The model under review builds one solid part; all positions refer to its coordinate system, in mm. A direction names the side the tool comes from. Round coordinates to 2 decimals unless told otherwise and drop trailing zeros. Order: outer loops, then holes, each group sorted by start corner. A loop starts at its lowest first (then second) coordinate and runs counter-clockwise, first axis right, second up.
```python
from build123d import *

# Parameters (mm, degrees)
SKETCH_1_W                = 42
SKETCH_1_H                = 30
EXTRUDE_1_DEPTH           = 40
CUT_EXTRUDE_1_DEPTH       = 85.059502735
HOLE_WIZARD_1_D           = 5.5
HOLE_WIZARD_1_CBORE_D     = 10
HOLE_WIZARD_1_CBORE_DEPTH = 23
CUT_EXTRUDE_2_DEPTH       = 85.059502735
HOLE_WIZARD_M8_1_D        = 6.8
HOLE_WIZARD_M8_1_DEPTH    = 19.75
HOLE_WIZARD_M8_1_TIP      = 2.042926105


with BuildPart() as part:
    # 草图1 → 凸台-拉伸1 (new, symmetric)
    with BuildSketch(Plane.XY):
        Rectangle(SKETCH_1_W, SKETCH_1_H)
    extrude(amount=EXTRUDE_1_DEPTH, both=True)

    # 草图2 → 切除-拉伸1 (cut, through all)
    with BuildSketch(Plane.XY.offset(40)):
        Polygon((-21, 12), (6, -15), (-21, -15), align=None)
    extrude(amount=-CUT_EXTRUDE_1_DEPTH, mode=Mode.SUBTRACT)

    # 打孔尺寸根据内六角圆柱头螺钉的类型1 (through all)
    with Locations(Plane(origin=(0, -15, 0), x_dir=(-1, 0, 0), z_dir=(0, -1, 0))):
        with Locations((0, -30), (0, 30), (0, 0)):
            CounterBoreHole(HOLE_WIZARD_1_D / 2, HOLE_WIZARD_1_CBORE_D / 2, HOLE_WIZARD_1_CBORE_DEPTH)

    # 草图3 → 切除-拉伸2 (cut, through all)
    with BuildSketch(Plane.XY.offset(40)):
        Polygon((-1.071067812, -7.928932188), (7.414213562, 0.556349186), (22.970562748, -15), (6, -15), align=None)
    extrude(amount=-CUT_EXTRUDE_2_DEPTH, mode=Mode.SUBTRACT)

    # M8 螺纹孔1
    with Locations(Plane(origin=(3.985281374, 3.985281374, 0), x_dir=(-0.7071067811865477, 0.7071067811865474, 0), z_dir=(-0.7071067811865474, -0.7071067811865477, 0))):
        with Locations((-12.849242405, 25), (-12.849242405, -25)):
            Hole(HOLE_WIZARD_M8_1_D / 2, depth=HOLE_WIZARD_M8_1_DEPTH)
            with Locations((0, 0, -(HOLE_WIZARD_M8_1_DEPTH + HOLE_WIZARD_M8_1_TIP / 2))):  # 118° drill point
                Cone(0, HOLE_WIZARD_M8_1_D / 2, HOLE_WIZARD_M8_1_TIP, mode=Mode.SUBTRACT)


solid = part.part
```
(1) Insertion check: pin 1 (8 mm diameter, centred on x = -2, z = -30.5, fed in from -Y); pin 2 (4.5 mm diameter, centred on x = 0, z = 30, fed in from +Y); pin 3 (11 mm diameter, centred on x = -1.5, z = 28, fed in from -Y); pin 4 (8 mm diameter, centred on y = 4.5, z = -25.5, fed in from +X). Each pin has a flat end and moves straight along its axis. Give the tip position at first contact, or say it passes through.
Data:
pin 1: stops at y = -6.81
pin 2: passes through
pin 3: stops at y = -7.93
pin 4: stops at x = 21
(2) Consider section C-C (z = 19). Write out the cut boundary in (x, y), and give its area (3 significant figures).
Data:
outline: (-21, 12) - (-1.07, -7.93) - (7.41, 0.56) - (21, -13.03) - (21, 15) - (-21, 15) - close
area: 705 mm2
(3) To check wall thickness, follow probe 1 along Z at (x, y) = (0, 11.75); probe 2 along Z at (x, y) = (0, 0); probe 3 along X at (y, z) = (12.25, -30). State the ranges of each line that lie inside material, in increasing order.
Data:
probe 1: z = -40 to -32.75, -27.25 to -2.75, 2.75 to 27.25, 32.75 to 40
probe 2: z = -40 to -35, -25 to -5, 5 to 25, 35 to 40
probe 3: x = -21 to -2.75, 2.75 to 21
(4) For faces 4 (the flat face through (-2.2, 8, 32.2)), 5 (the cylindrical face through (-0.596, 11.549, 2.685)), 6 (the flat face through (5.94, -0.92, 0.56)), list the 3-axis set-ups (+Z, -Z, +X, -X, +Y, -Y) from which the entire face can be reached by the end or side of a thin tool; tool diameter is ignored.
Data:
face 4: -Y
face 5: +Y, -Y
face 6: +Z, -Z, -Y
(5) Draft analysis for pull direction X (two halves, no side actions). For faces 1 (the flat face through (-2.2, 8, -27.8)), 2 (the flat face through (-5, 15, 1)), 3 (the flat face through (21, 1, 1)), state which applies: pulls with the +X half, pulls with the -X half, needs draft (parallel to the pull), parting line crosses it, or undercut.
Data:
face 1: undercut
face 2: needs draft
face 3: pulls with the +X half
(6) Consider section A-A (z = 30). Write out the cut boundary in (x, y).
Data:
outline: (-21, 12) - (-5, -4) - (-5, 8) - (-2.75, 8) - (-2.75, 15) - (-21, 15) - close; (2.75, 8) - (5, 8) - (5, -1.86) - (7.41, 0.56) - (21, -13.03) - (21, 15) - (2.75, 15) - close
(7) Consider section D-D (x = -8). Write out the cut boundary in (y, z).
Data:
outline: (-1, -40) - (15, -40) - (15, 40) - (-1, 40) - close
(8) Consider section B-B (y = -0.5). State how many separate pieces and enclosed holes the cut face has, and give its area (3 significant figures).
Data:
separate pieces: 2
enclosed holes: 3
area: 1,860 mm2
